```python
from build123d import *

# Parameters (mm, degrees)
BOSS_EXTRU_1_DEPTH      = 1500
ENL_V_MAT_EXTRU_1_DEPTH = 1507.651917332
ESQUISSE5_R             = 23.5
ENL_V_MAT_EXTRU_2_DEPTH = 1507.651917332
ESQUISSE6_W             = 100
ESQUISSE6_H             = 129
ENL_V_MAT_EXTRU_3_DEPTH = 1507.651917332


with BuildPart() as part:
    # Esquisse2 → Boss.-Extru.1 (new body)
    with BuildSketch(Plane(origin=(0, 0, 0), x_dir=(1, 0, 0), z_dir=(0, 1, 0))):
        with BuildLine():
            Line((2, 0), (98, 0))
            ThreePointArc((98, 0), (99.414213562, 0.585786438), (100, 2))
            Line((100, 2), (100, 98))
            ThreePointArc((100, 98), (99.414213562, 99.414213562), (98, 100))
            Line((98, 100), (2, 100))
            ThreePointArc((2, 100), (0.585786438, 99.414213562), (0, 98))
            Line((0, 98), (0, 2))
            ThreePointArc((0, 2), (0.585786438, 0.585786438), (2, 0))
        make_face()
        with BuildLine():
            Line((6, 96), (94, 96))
            ThreePointArc((94, 96), (95.414213562, 95.414213562), (96, 94))
            Line((96, 94), (96, 6))
            ThreePointArc((96, 6), (95.414213562, 4.585786438), (94, 4))
            Line((94, 4), (6, 4))
            ThreePointArc((6, 4), (4.585786438, 4.585786438), (4, 6))
            Line((4, 6), (4, 94))
            ThreePointArc((4, 94), (4.585786438, 95.414213562), (6, 96))
        make_face(mode=Mode.SUBTRACT)
    extrude(amount=BOSS_EXTRU_1_DEPTH)

    # Esquisse4 → Enlèv. mat.-Extru.1 (cut, through all)
    with BuildSketch(Plane.ZY):
        Polygon((0, 200), (-206.800963523, -46.455791231), (114.552024245, -46.455791231), (114.552024245, 200), align=None)
    extrude(amount=-ENL_V_MAT_EXTRU_1_DEPTH, mode=Mode.SUBTRACT)

    # Esquisse5 → Enlèv. mat.-Extru.2 (cut, through all)
    with BuildSketch(Plane(origin=(0, 0, -100), x_dir=(-1, 0, 0), z_dir=(0, 0, -1))):
        with Locations((-50, 1271)):
            Circle(ESQUISSE5_R)
    extrude(amount=-ENL_V_MAT_EXTRU_2_DEPTH, mode=Mode.SUBTRACT)

    # Esquisse6 → Enlèv. mat.-Extru.3 (cut, through all)
    with BuildSketch(Plane(origin=(0, 0, -100), x_dir=(-1, 0, 0), z_dir=(0, 0, -1))):
        with Locations((-50, 1435.5)):
            Rectangle(ESQUISSE6_W, ESQUISSE6_H)
    extrude(amount=-ENL_V_MAT_EXTRU_3_DEPTH, mode=Mode.SUBTRACT)


solid = part.part
```
Model file for the job. Use its own axes, mm. A direction names the side the tool comes from. Coordinates: 2 decimals unless noted, no trailing zeros. Loops run counter-clockwise (first coordinate to the right, second up) from the corner with the lowest first, then second, coordinate; pieces in that order, holes last. Notation, with made-up numbers: (28, -35.5) - (78, -35.5) arc R20 cw to (78, -29.5) - close; hole circle Ø2 at (78, -17.75). An arc over 180 degrees is marked (long way). Write item = value, one per line. Start each with the question number.
Item 1: 3-axis set-ups, long thin cutter, end or side, ignore diameter. For faces 4 (the face through (49, 777, 0)), 5 (the face through (49, 719, -96)): which of +Z, -Z, +X, -X, +Y, -Y reach the whole face in a straight line?
Item 2: Pull direction Y, two halves, no side cores. Call faces 1 (the face through (54, 1371, -2)), 2 (the face through (51, 775, -4)), 3 (the face through (53.06, 1294.3, -2.03)): +Y half, -Y half, draft (parallel to the pull), parting line (faces both ways), or undercut.
Item 3: Saw through at A-A, the plane y = 1271. List the corners of the cut face in (x, z), then the cut area to 3 significant figures.
Item 4: Saw through at D-D, the plane z = -61.5. List the corners of the cut face in (x, y), then the cut area to 3 significant figures.
Item 5: Wall check: probe 1 along Z at (x, y) = (10.5, 263); probe 2 along Y at (x, z) = (50, -98.1); probe 3 along X at (y, z) = (408, -63.5). Give the ranges that are in metal, low to high. Write a range as [from, to].
Item 6: Saw through at B-B, the plane x = 50. List the corners of the cut face in (y, z).
Item 7: Saw through at C-C, the plane y = 1066.5. List the corners of the cut face in (x, z).
Item 8: Drop a flat-ended pin along its axis: pin 1 Ø12 at (x, z) = (85, -79) entering from -Y. Give the stop position or say it passes through.
Answers:
q1.face_4 = +Z, +X, -X, +Y, -Y
q1.face_5 = +Y, -Y
q2.face_1 = +Y half
q2.face_2 = draft
q2.face_3 = undercut
q3.outline = (0, -98) arc R2 ccw to (2, -100) - (26.5, -100) - (26.5, -96) - (6, -96) arc R2 cw to (4, -94) - (4, -6) arc R2 cw to (6, -4) - (26.5, -4) - (26.5, 0) - (2, 0) arc R2 ccw to (0, -2) - close; (73.5, -100) - (98, -100) arc R2 ccw to (100, -98) - (100, -2) arc R2 ccw to (98, 0) - (73.5, 0) - (73.5, -4) - (94, -4) arc R2 cw to (96, -6) - (96, -94) arc R2 cw to (94, -96) - (73.5, -96) - close
q3.area = 1,160 mm2
q4.outline = (0, 126.71) - (4, 126.71) - (4, 1371) - (0, 1371) - close; (96, 126.71) - (100, 126.71) - (100, 1371) - (96, 1371) - close
q4.area = 9,950 mm2
q5.probe_1 = [-100, -96], [-4, 0]
q5.probe_2 = [83.09, 1247.5], [1294.5, 1371]
q5.probe_3 = [0, 4], [96, 100]
q6.outline = (80.82, -100) - (1247.5, -100) - (1247.5, -96) - (85.59, -96) - close; (195.23, -4) - (1247.5, -4) - (1247.5, 0) - (200, 0) - close; (1294.5, -100) - (1371, -100) - (1371, -96) - (1294.5, -96) - close; (1294.5, -4) - (1371, -4) - (1371, 0) - (1294.5, 0) - close
q7.outline = (0, -98) arc R2 ccw to (2, -100) - (98, -100) arc R2 ccw to (100, -98) - (100, -2) arc R2 ccw to (98, 0) - (2, 0) arc R2 ccw to (0, -2) - close; hole (4, -94) arc R2 ccw to (6, -96) - (94, -96) arc R2 ccw to (96, -94) - (96, -6) arc R2 ccw to (94, -4) - (6, -4) arc R2 ccw to (4, -6) - close
q8.pin_1 = through
